```python
from build123d import *

# Parameters (mm, degrees)
WYCI_GNI_CIE_CIENKA_CIANKA2_DEPTH      = 170
WYCI_GNI_CIE_CIENKA_CIANKA2_DEPTH_BACK = 170
WYTNIJ_WYCI_GNI_CIE2_START             = -10
SZKIC3_R                               = 5
WYTNIJ_WYCI_GNI_CIE2_DEPTH             = 50


with BuildPart() as part:
    # Szkic2 → Wyciągnięcie-cienka ścianka2 (new, two sides: drawn at the far end of the back side and taken through both)
    with BuildSketch(Plane(origin=(0, 0, 0), x_dir=(0, 0, -1), z_dir=(1, 0, 0)).offset(-WYCI_GNI_CIE_CIENKA_CIANKA2_DEPTH_BACK)):
        Polygon((0, 50), (0, 0), (-12.5, -21.650635095), (-12.5, -71.650635095), (-15.5, -71.650635095), (-15.5, -20.846787517), (-3, 0.803847577), (-3, 50), align=None)
    extrude(amount=WYCI_GNI_CIE_CIENKA_CIANKA2_DEPTH + WYCI_GNI_CIE_CIENKA_CIANKA2_DEPTH_BACK)

    # Szkic3 → Wytnij-wyciągnięcie2 (cut)
    with BuildSketch(Plane.XY.offset(3).offset(WYTNIJ_WYCI_GNI_CIE2_START)):
        with Locations(Location((-135.725, 25.401923789, 0), (0, 0, 270))):
            Circle(SZKIC3_R)
        with Locations(Location((-135.725, -51.650635095, 0), (0, 0, 270))):
            Circle(SZKIC3_R)
    wytnij_wyci_gni_cie2 = extrude(amount=WYTNIJ_WYCI_GNI_CIE2_DEPTH, mode=Mode.SUBTRACT)

    # Lustro1: Wytnij-wyciągnięcie2 across plane
    add(wytnij_wyci_gni_cie2.mirror(Plane(origin=(0, 0, 0), x_dir=(0, 0, 1), z_dir=(1, 0, 0))), mode=Mode.SUBTRACT)


solid = part.part
```
Can you work these out from the model? Positions are in its coordinate system, mm. A direction names the side the tool comes from. Round coordinates to 2 decimals unless told otherwise and drop trailing zeros. Loops run counter-clockwise (first coordinate to the right, second up) from the corner with the lowest first, then second, coordinate; pieces in that order, holes last.
Item 1: Suppose I cut it at B-B, the plane x = 52.5. Write out the boundary of the cut face in (y, z).
Item 2: Suppose I cut it at C-C, the plane z = 6.75. Write out the boundary of the cut face in (x, y).
Item 3: If we mould it in two halves opening along Y, with no side actions, what happens to faces 1 (the cylindrical face through (-140.606, -50.567, 13.979)), 2 (the flat face through (-2.38, -10.67, 6.16)), 3 (the cylindrical face through (140.606, -50.567, 13.979)), 4 (the flat face through (-2, -47, 15.5))? For each: +Y half, -Y half, draft (parallel to the pull), parting line (faces both ways), or undercut.
Item 4: Will these pins go through, and if not, where does the flat tip stop? pin 1 Ø5 at (x, z) = (-2.5, 4.5) entering from +Y; pin 2 Ø24.5 at (x, y) = (-47.5, 29.5) entering from +Z; pin 3 Ø15 at (x, y) = (-46.5, -39) entering from -Z; pin 4 Ø10 at (x, y) = (-135, -7) entering from +Z.
Item 5: Suppose I cut it at D-D, the plane y = 4. Write out the boundary of the cut face in (x, z).
Item 6: Suppose I cut it at A-A, the plane y = 24.5. Write out the boundary of the cut face in (x, z), then the cut area to 3 significant figures.
Item 7: Which directions (+Z, -Z, +X, -X, +Y, -Y) give clear straight access to the entire face, cutting with the end or side of a thin tool? Please do faces 5 (the cylindrical face through (-140.606, 26.486, 1.479)), 6 (the flat face through (-2, -46, 12.5)), 7 (the flat face through (-2, 25, 3)).
Item 8: Please list where these lines run through material, in increasing order: L1, parallel to Z at x = -39, y = -50; L2, parallel to Z at x = -16, y = 13.5; L3, parallel to X at y = -49, z = 14.
Reported:
1. outline: (-71.65, 12.5) - (-21.65, 12.5) - (0, 0) - (50, 0) - (50, 3) - (0.8, 3) - (-20.85, 15.5) - (-71.65, 15.5) - close
2. outline: (-170, -11.69) - (170, -11.69) - (170, -5.69) - (-170, -5.69) - close
3. face 1: undercut
3. face 2: -Y half
3. face 3: undercut
3. face 4: draft
4. pin 1: stops at y = 50
4. pin 2: stops at z = 3
4. pin 3: stops at z = 12.5
4. pin 4: stops at z = 10.39
5. outline: (-170, 0) - (170, 0) - (170, 3) - (-170, 3) - close
6. outline: (-170, 0) - (-140.64, 0) - (-140.64, 3) - (-170, 3) - close; (-130.81, 0) - (130.81, 0) - (130.81, 3) - (-130.81, 3) - close; (140.64, 0) - (170, 0) - (170, 3) - (140.64, 3) - close
6. area: 961 mm2
7. face 5: +Z, -Z
7. face 6: -Z, +X, -X, -Y
7. face 7: +Z, +X, -X, +Y
8. L1: z = 12.5 to 15.5
8. L2: z = 0 to 3
8. L3: x = -170 to -139.96, -131.49 to 131.49, 139.96 to 170
